Could you check a few things on this model? Use its own coordinates, in mm. Face numbers are marked on the shaded views. A direction names the side the tool comes from. Round coordinates to 2 decimals unless told otherwise and drop trailing zeros. Loops run counter-clockwise (first coordinate to the right, second up) from the corner with the lowest first, then second, coordinate; pieces in that order, holes last. Notation, with made-up numbers: (4, -6.75) -> (29, -6.75) arc R9 cw to (29, 7.25) -> close; hole circle Ø9 at (52.25, -25). An arc over 180 degrees is marked (long way). One line per item, written item: value.
Autodesk Inventor part; units mm, degrees
ref_plane "YZ Plane" through (0, 0, 0) normal (1, 0, 0) x (0, 1, 0)
ref_plane "XZ Plane" through (0, 0, 0) normal (0, 1, 0) x (-1, 0, 0)
ref_plane "XY Plane" through (0, 0, 0) normal (0, 0, 1) x (1, 0, 0)
ref_plane "Work Plane1" through (0, 0, 0) normal (0, 0, 1) x (1, 0, 0)
sketch "Sketch1" plane through (0, 0, 0) normal (0, 0, 1) x (1, 0, 0)
  line L0 (0, 0) -> (21, 0)
  line L1 (15.5, 0) -> (15.5, -20)
  circle A0 centre (0, 0) radius 15.5
  line L2 (0, 0) -> (14.0478, -6.5506)
  line L3 (0, 0) -> (0, -16.875)
  line L4 (0, 0) -> (-18.25, 0)
  line L5 (0, 0) -> (0, 19.625)
  arc A1 (-18.25, 0) -> (15.5, 0) centre (-1.375, -0.056) ccw
  arc A2 (21, 0) -> (-18.25, 0) centre (1.375, 0.0482) ccw
  line L6 (21, 0) -> (21, -20)
  line L7 (0, 0) -> (0, -18.875)
  line L8 (0, 0) -> (-20.25, 0)
  line L9 (0, 0) -> (0, 21.625)
  line L10 (0, 0) -> (23, 0)
  line L11 (0, 0) -> (17.5, 0)
  arc A3 (-20.25, 0) -> (17.5, 0) centre (-1.375, -0.0501) ccw
  arc A4 (23, 0) -> (-20.25, 0) centre (1.375, 0.0437) ccw
  line L12 (13.5, -8.0249) -> (13.5, -20)
  line L13 (15.5, -20) -> (13.5, -20)
  line L14 (23, 0) -> (23, -20)
  line L15 (21, -20) -> (23, -20)
  line L16 (21, -20) -> (15.5, -20)
  point P0 (15.5, -8.506)
  point P1 (15.5, -0.112)
  point P2 (21, 0)
  point P3 (13.5, -14.0125)
  point P4 (13.5, -11.6691)
  dimension "d2" = 31
  dimension "d0" = 21
  dimension "d1" = 15.5
  dimension "d3" = 25
  dimension "d4" = 16.875
  dimension "d5" = 18.25
  dimension "d6" = 19.625
  dimension "d7" = 20
  dimension "d8" = 20
  dimension "d9" = 2
  dimension "d10" = 2
  dimension "d11" = 2
  dimension "d12" = 2
  dimension "d13" = 2
  dimension "d16" = 2
extrude "Extrusion1" add sketch "Sketch1" along normal blind 18 contours L1 A3 L12 A1 | L1 L13 L12 A3 | L12 A3 L7 A1 | L7 A3 L8 A1 | L8 A4 L9 A2 | L9 A4 L10 A2 | L10 L14 L15 L6
extrude "Extrusion2" add sketch "Sketch1" along normal blind 3 contours L5 A0 L0 | L0 A0 L2 | L2 A0 L3 | L3 A0 L4 | L4 A0 L5 | A0 L5 A2 L0 | L0 A3 L1 | A1 L3 A0 | L3 A1 L4 A0 | L4 A2 L5 A0 | L0 L6 L16 L1 A3
sketch "Sketch2" plane through (13.5, -20, 0) normal (0, -1, 0) x (1, 0, 0)
  circle A0 centre (4.7788, 10.8992) radius 2.75
  point P0 (-13.5, 0)
  dimension "d19" = 5.5
equation "\"d2\" = VoluteCaseInnerSize"
equation "\"d0\" = 0.5 * VoluteCaseOuterSize"
equation "\"d1\" = 0.5 * VoluteCaseInnerSize"
equation "\"d3\" = VoluteStartAngle"
equation "\"d4\" = 0.375 * VoluteCaseInnerSize + 0.125 * VoluteCaseOuterSize"
equation "\"d5\" = 0.25 * VoluteCaseInnerSize + 0.25 * VoluteCaseOuterSize"
equation "\"d6\" = 0.125 * VoluteCaseInnerSize + 0.375 * VoluteCaseOuterSize"
equation "\"d7\" = VoluteOutletLength"
equation "\"d8\" = VoluteOutletLength"
equation "\"d9\" = VoluteWallThickness"
equation "\"d10\" = VoluteWallThickness"
equation "\"d11\" = VoluteWallThickness"
equation "\"d12\" = VoluteWallThickness"
equation "\"d13\" = VoluteWallThickness"
equation "\"d14\" = VoluteBaseWallThickness + VoluteWallDepth"
equation "\"d17\" = VoluteBaseWallThickness"
equation "\"d19\" = OutletRadius"
equation "\"PropHoleDiameter\" = 8.2"
equation "\"PropBladeThickness\" = 1"
equation "\"PropPlateThickness\" = 2"
equation "\"VoluteCaseInnerSize\" = 31"
equation "\"VoluteCaseOuterSize\" = 42"
equation "\"VoluteWallThickness\" = 2"
equation "\"VoluteStartAngle\" = 25deg"
equation "\"VoluteOutletLength\" = 20"
equation "\"VoluteBaseWallThickness\" = 3"
equation "\"VoluteWallDepth\" = 15"
equation "\"OutletRadius\" = 5.5"
properties part number "volute_case"
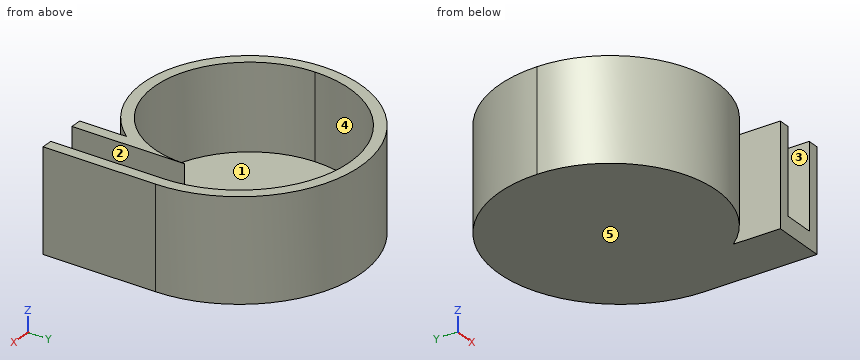
(1) On a 3-axis mill with a long thin cutter (end or side, diameter ignored), from which of +Z, -Z, +X, -X, +Y, -Y can I reach the whole of each face in a straight line? I mean the marked faces 3, 4 and 5. Say none if no direction works.
Results below:
face 3: +Z, -Y
face 4: +Z
face 5: -Z, +X, -X, +Y, -Y
(2) We'd pull the mould along Y, two halves only. Please class the marked faces 1 and 2: +Y half, -Y half, draft (parallel to the pull), parting line (faces both ways), or undercut.
Results below:
face 1: undercut
face 2: draft
(3) Imagine slicing it at A-A on y = -16. Write out the boundary of the cut face in (x, z), then the cut area to 3 significant figures.
Results below:
outline: (-11.47, 0) -> (8.72, 0) -> (8.72, 18) -> (4.15, 18) -> (4.15, 3) -> (-6.9, 3) -> (-6.9, 18) -> (-11.47, 18) -> close; (13.5, 0) -> (23, 0) -> (23, 18) -> (21, 18) -> (21, 3) -> (15.5, 3) -> (15.5, 18) -> (13.5, 18) -> close
area: 286 mm²
(4) For pin 1 Ø6 at (y, z) = (6, 4.5) entering from -X; pin 2 Ø1.5 at (x, y) = (-3, 11.5) entering from +Z; pin 3 Ø10 at (x, z) = (-6.5, 11) entering from -Y, each with a flat end and sliding along its axis, tell me the tip position at first contact or that it passes through.
Results below:
pin 1: stops at x = -20.05
pin 2: stops at z = 3
pin 3: stops at y = -18.92
(5) Imagine slicing it at C-C on z = 9. Write out the boundary of the cut face in (x, y) (3 decimals).
Results below:
outline: (-20.25, 0) arc R18.875 ccw to (13.5, -11.669) -> (13.5, -20) -> (15.5, -20) -> (15.5, -0.112) arc R16.875 cw to (-18.25, 0) arc R19.625 cw to (21, 0) -> (21, -20) -> (23, -20) -> (23, 0) arc R21.625 ccw to start
(6) Imagine slicing it at D-D on y = -2. Write out the boundary of the cut face in (x, z), then the cut area to 3 significant figures.
Results below:
outline: (-20.15, 0) -> (23, 0) -> (23, 18) -> (21, 18) -> (21, 3) -> (15.5, 3) -> (15.5, 18) -> (15.39, 18) -> (15.39, 3) -> (-18.14, 3) -> (-18.14, 18) -> (-20.15, 18) -> close
area: 191 mm²
(7) Please list where these lines run through material, in increasing order: L1, parallel to X at y = -15, z = 15; L2, parallel to Z at x = -16.5, y = 1; L3, parallel to Y at x = -14.5, z = 8.25.
Results below:
L1: x = -12.9 to -9.21, 6.46 to 10.15, 13.5 to 15.5, 21 to 23
L2: z = 0 to 3
L3: y = -13.61 to -10.66, 11.59 to 14.73
(8) Imagine slicing it at B-B on x = -0.5. Write out the boundary of the cut face in (y, z).
Results below:
outline: (-18.9, 0) -> (21.59, 0) -> (21.59, 18) -> (19.58, 18) -> (19.58, 3) -> (-16.91, 3) -> (-16.91, 18) -> (-18.9, 18) -> close
